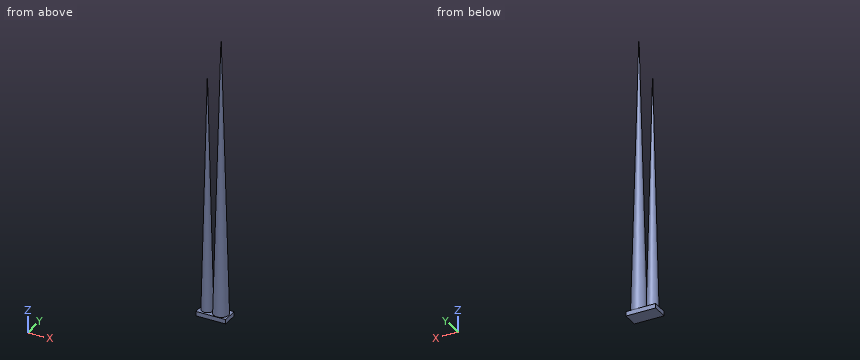
Solid Edge part; units mm, degrees
sketch "Sketch1" plane through (0, 0, 0) normal (0, 0, 1) x (1, 0, 0)
  line L0 (0, 0) -> (105, 0)
  line L1 (105, 0) -> (105, 55)
  line L2 (105, 55) -> (0, 55)
  line L3 (0, 55) -> (0, 0)
extrude "Protrusion1" add sketch "Sketch1" against normal blind 16
sketch "Sketch2" plane through (52.5, 27.5, -8) normal (0, -1, 0) x (1, 0, 0)
  line L0 (-26.8767, 858) -> (-6.7387, 8)
  line L1 (-6.7387, 8) -> (-26.8767, 8)
  line L2 (-26.8767, 8) -> (-26.8767, 858)
revolve "RevolvedProtrusion1" add sketch "Sketch2" angle 360 about axis through (25.6233, 27.5, 0) along (0, 0, 1)
sketch "Sketch3" plane through (52.5, 27.5, -8) normal (0, -1, 0) x (1, 0, 0)
  line L0 (21.4521, 1008) -> (47.7271, 8)
  line L1 (47.7271, 8) -> (21.4521, 8)
  line L2 (21.4521, 8) -> (21.4521, 1008)
revolve "RevolvedProtrusion2" add sketch "Sketch3" angle 360 about axis through (73.9521, 27.5, 0) along (0, 0, 1)
Here's how the part is built. I have some questions about the finished solid (model axes, mm). Round coordinates to 2 decimals unless told otherwise and drop trailing zeros. Loops run counter-clockwise (first coordinate to the right, second up) from the corner with the lowest first, then second, coordinate; pieces in that order, holes last.
1. If we section it at A-A on z = 595: Write out the boundary of the cut face in (x, y).
Answer list:
outline: circle Ø12.08 at (25.62, 27.5); circle Ø21.28 at (73.95, 27.5)
2. If we section it at B-B on z = 778: Write out the boundary of the cut face in (x, y), plus the area to 3 significant figures.
Answer list:
outline: circle Ø3.41 at (25.62, 27.5); circle Ø11.67 at (73.95, 27.5)
area: 116 mm2
3. If I drill on line 1 along Z through (x, y) = (54, 52); line 2 along X through (y, z) = (39, 109); line 3 along X through (y, z) = (27, 168), over which ranges is the centre line in solid material (lowest first)?
Answer list:
line 1: z = -16 to 0
line 2: x = 12.36 to 38.89, 53.56 to 94.34
line 3: x = 9.47 to 41.77, 52.1 to 95.81
4. For P1, Ø10, axis at x = 93, z = 556.5, coming from the +Y side; P2, Ø6, axis at x = 63.5, z = 327.5, coming from the -Y side; P3, Ø5, axis at x = 33, z = 484, coming from the -Y side; P4, Ø2, axis at y = 33.5, z = 463.5, coming from the -X side, each with a flat end and sliding along its axis, tell me the tip position at first contact or that it passes through.
Answer list:
P1: passes through
P2: stops at y = 11.48
P3: stops at y = 20.33
P4: stops at x = 17.95
